The model under review builds one solid part; all positions refer to its coordinate system, in mm. A direction names the side the tool comes from. Coordinates: 2 decimals unless noted, no trailing zeros. Loops run counter-clockwise (first coordinate to the right, second up) from the corner with the lowest first, then second, coordinate; pieces in that order, holes last. Notation, with made-up numbers: (13, -5) - (52, -5) arc R18 cw to (52, 4) - close; hole circle Ø6 at (80, 27). An arc over 180 degrees is marked (long way). One line per item, written item: value. Start each with the question number.
1. We need section D-D, the plane x = 6. Give the boundary of the cut face in (y, z), then the cut area to 3 significant figures.
2. We need section C-C, the plane y = -29.5. Give the boundary of the cut face in (x, z), then the cut area to 3 significant figures.
3. To check wall thickness, follow line 1 (Y direction, x = 0, z = 2); line 2 (X direction, y = 21, z = 2.85); line 3 (Y direction, x = 1, z = 0.35). State the ranges of each line that lie inside material, in increasing order.
4. Insertion check: P1, Ø1.5, axis at y = 10, z = 2, coming from the -X side; P2, Ø1.5, axis at y = 36, z = 1.5, coming from the +X side. Each pin has a flat end and moves straight along its axis. Give the tip position at first contact, or say it passes through.
5. We need section A-A, the plane y = 0. Give the boundary of the cut face in (x, z), then the cut area to 3 significant figures.
6. For faces 1 (the face through (2, -36, 1)), 2 (the face through (-2, 31, 1)), 3 (the face through (0, -4, 3)), 4 (the face through (-2, -37, 1)), list the 3-axis set-ups (+Z, -Z, +X, -X, +Y, -Y) from which the entire face can be reached by the end or side of a thin tool; tool diameter is ignored.
7. Mouldability with a two-part tool opening along Y and no side actions: class faces 5 (the face through (2.484, 7.609, 1.521)), 6 (the face through (-2.579, 1.978, 1.479)), 7 (the face through (2, 32, 1)) as +Y half, -Y half, draft (parallel to the pull), parting line (faces both ways), or undercut.
Autodesk Fusion 360 part; units mm, degrees
sketch "Mixer arm" plane through (0, 0, 0) normal (0, 0, 1) x (1, 0, 0)
  circle A0 centre (0, 0) radius 7.25
  circle A1 centre (0, 0) radius 3.25
  line L0 (-2, 55.25) -> (2, 55.25)
  line L1 (2, 55.25) -> (2, 3.25)
  line L2 (2, 3.25) -> (-2, 3.25)
  line L3 (-2, 3.25) -> (-2, 55.25)
  line L4 (-2, -3.25) -> (2, -3.25)
  line L5 (2, -3.25) -> (2, -65.25)
  line L6 (2, -65.25) -> (-2, -65.25)
  line L7 (-2, -65.25) -> (-2, -3.25)
  line L8 (-2, -7.25) -> (2, -7.25)
  line L9 (-2, 7.25) -> (2, 7.25)
  dimension "d3" = 6.5
  dimension "d5" = 14.5
  dimension "d6" = 2
  dimension "d7" = 2
  dimension "d8" = 2
  dimension "d9" = 2
  dimension "d14" = 58
  dimension "d15" = 48
extrude "Extrude1" add sketch "Mixer arm" along normal blind 3 contours A0 A1 L1 L2 L4 L5 | A0 L1 L2 L3 | A0 L1 L9 | A0 L5 L8 | A0 L4 L5 L7 | A0 L3 L9 | L0 L1 L3 L9 | A0 L7 L8 | L5 L6 L7 L8 | A0 A1 L2 L3 L4 L7
fillet "Fillet1" radius 4 4 edges at (2, -6.9687, 1.5) (2, 6.9687, 1.5) (-2, 6.9687, 1.5) (-2, -6.9687, 1.5)
fillet "Fillet2" radius 2 4 edges at (2, 55.25, 1.5) (-2, 55.25, 1.5) (-2, -65.25, 1.5) (2, -65.25, 1.5)
equation "stainless_steel_thickness = 3 mm"
equation "hole_diameter = 6.5 mm"
equation "d3 = hole_diameter"
equation "arm_thickness = 4 mm"
equation "d5 = hole_diameter + 2 * arm_thickness"
equation "d6 = arm_thickness / 2"
equation "d7 = arm_thickness / 2"
equation "d8 = arm_thickness / 2"
equation "d9 = arm_thickness / 2"
equation "d10 = stainless_steel_thickness"
equation "arm_length_front = 58 mm"
equation "arm_length_back = 48 mm"
equation "d14 = arm_length_front"
equation "d15 = arm_length_back"
equation "d17 = arm_thickness"
equation "d19 = arm_thickness / 2"
Findings below:
1. outline: (-4.07, 0) - (4.07, 0) - (4.07, 3) - (-4.07, 3) - close
1. area: 24.4 mm2
2. outline: (-2, 0) - (2, 0) - (2, 3) - (-2, 3) - close
2. area: 12.0 mm2
3. line 1: -65.25 to -3.25, 3.25 to 55.25
3. line 2: -2 to 2
3. line 3: -64.98 to -3.09, 3.09 to 54.98
4. P1: x = -2.01
4. P2: x = 2
5. outline: (-7.25, 0) - (-3.25, 0) - (-3.25, 3) - (-7.25, 3) - close; (3.25, 0) - (7.25, 0) - (7.25, 3) - (3.25, 3) - close
5. area: 24.0 mm2
6. face 1: +Z, -Z, +X, -Y
6. face 2: +Z, -Z, -X, +Y
6. face 3: +Z, +X, -X, +Y, -Y
6. face 4: +Z, -Z, -X, -Y
7. face 5: +Y half
7. face 6: undercut
7. face 7: draft
